Geometry check sheet. Reference: the model listing, model coordinates, mm. A direction names the side the tool comes from. Give positions to 0.01 mm unless a question says otherwise; leave off trailing zeros. Order: outer loops, then holes, each group sorted by start corner. A loop starts at its lowest first (then second) coordinate and runs counter-clockwise, first axis right, second up.
from build123d import *

# Parameters (mm, degrees)
F0_W     = 612
F0_H     = 40
F1_DEPTH = 628
F2_W     = 612
F2_H     = 100
F3_DEPTH = 25


with BuildPart() as f1:
    # F0 (on Front) → F1 (new body)
    with BuildSketch(Plane.XZ):
        Rectangle(F0_W, F0_H)
    extrude(amount=F1_DEPTH)

    # F2 (on face) → F3 (join)
    with BuildSketch(Plane(origin=(0, 0, 0), x_dir=(-1, 0, 0), z_dir=(0, 1, 0))):
        with Locations((0, 70)):
            Rectangle(F2_W, F2_H)
    extrude(amount=-F3_DEPTH)


solid = f1.part
Item 1: Scan lines: L1, parallel to Z at x = -9.5, y = -558; L2, parallel to Y at x = 34, z = 35.5. Record each from-to range of solid material in increasing order.
Reported:
L1: z = -20 to 20
L2: y = -25 to 0
Item 2: Set-up check for faces 1 (the flat face through (-4, -322, 20)), 2 (the flat face through (306, -289, 8)): record each of +Z, -Z, +X, -X, +Y, -Y from which the full face is reachable in a straight line by a thin tool's end or side.
Reported:
face 1: +Z, +X, -X, -Y
face 2: +Z, -Z, +X, +Y, -Y
Item 3: Sectioned sample at A-A (x = -67.5). Enter the section's corners in (y, z).
Reported:
outline: (-628, -20) - (0, -20) - (0, 120) - (-25, 120) - (-25, 20) - (-628, 20) - close
Item 4: Sectioned sample at B-B (y = -322.5). Enter the section's corners in (x, z).
Reported:
outline: (-306, -20) - (306, -20) - (306, 20) - (-306, 20) - close
Item 5: Gauge pin test, flat ends, axial feed: pin 1 (1 mm diameter, centred on x = 179, z = 14.5, fed in from +Y); pin 2 (5 mm diameter, centred on x = -8, y = -100.5, fed in from +Z); pin 3 (10 mm diameter, centred on x = 157, z = 42.5, fed in from -Y). Record the tip position at first contact, or that the pin passes through.
Reported:
pin 1: stops at y = 0
pin 2: stops at z = 20
pin 3: stops at y = -25
Item 6: Sectioned sample at C-C (z = 94). Enter the section's corners in (x, y).
Reported:
outline: (-306, -25) - (306, -25) - (306, 0) - (-306, 0) - close
